Read the model definition and answer for the solid it produces. Units are mm, in the model's axes. A direction names the side the tool comes from. Coordinates: 2 decimals unless noted, no trailing zeros. Write each loop counter-clockwise with the first axis right and the second up, starting at its lowest first coordinate (ties: lowest second). Pieces come first, ordered by that corner, then holes. Notation, with made-up numbers: (-18, -39) - (-12, -39) arc R21 cw to (-12, -22) - close; hole circle Ø2 at (18, 82.5). An arc over 180 degrees is marked (long way). Return JSON: item names as keys, results as strings.
```python
from build123d import *

# Parameters (mm, degrees)
SKETCH_1_W          = 160
SKETCH_1_H          = 70
EXTRUDE_1_DEPTH     = 180
SHELL_1_T           = -10
SKETCH_2_W          = 3
SKETCH_2_H          = 70
EXTRUDE_2_DEPTH     = 170
CUT_EXTRUDE_1_DEPTH = 170
CUT_EXTRUDE_2_DEPTH = 170
CUT_EXTRUDE_3_REACH = 245.362
SKETCH_6_W          = 160
SKETCH_6_H          = 10
EXTRUDE_3_DEPTH     = 10
FILLET_1_R          = 3


with BuildPart() as part:
    # 草图1 → 凸台-拉伸1 (new body)
    with BuildSketch(Plane(origin=(0, 0, 0), x_dir=(1, 0, 0), z_dir=(0, 1, 0))):
        Rectangle(SKETCH_1_W, SKETCH_1_H)
    extrude(amount=EXTRUDE_1_DEPTH)

    # 抽壳1
    shell_1_openings = [part.faces().sort_by_distance(p)[0] for p in [
        (0, 90, 35),
    ]]
    offset(amount=SHELL_1_T, openings=shell_1_openings, kind=Kind.INTERSECTION)

    # 草图2 → 凸台-拉伸2 (add)
    with BuildSketch(Plane.XZ):
        with Locations((31.5, 0)):
            Rectangle(SKETCH_2_W, SKETCH_2_H)
        with Locations((28.5, 0)):
            Rectangle(SKETCH_2_W, SKETCH_2_H)
    extrude(amount=-EXTRUDE_2_DEPTH)

    # 草图3 → 切除-拉伸1 (cut)
    with BuildSketch(Plane.XY.offset(-25)):
        with BuildLine():
            Line((-8, 140), (-8, 40))
            ThreePointArc((-8, 40), (-21.5, 26.5), (-35, 40))
            Line((-35, 40), (-35, 140))
            ThreePointArc((-35, 140), (-21.5, 153.5), (-8, 140))
        make_face()
    extrude(amount=-CUT_EXTRUDE_1_DEPTH, mode=Mode.SUBTRACT)

    # 草图4 → 切除-拉伸2 (cut)
    with BuildSketch(Plane.XY.offset(-25)):
        with BuildLine():
            Line((59, 137.5), (59, 42.5))
            ThreePointArc((59, 42.5), (51.5, 35), (44, 42.5))
            Line((44, 42.5), (44, 137.5))
            ThreePointArc((44, 137.5), (51.5, 145), (59, 137.5))
        make_face()
    extrude(amount=-CUT_EXTRUDE_2_DEPTH, mode=Mode.SUBTRACT)

    # 草图5 → 切除-拉伸3 (cut, up to next)
    with BuildSketch(Plane.ZY.offset(80), mode=Mode.PRIVATE) as cut_extrude_3_sk1:
        with BuildLine():
            Line((-9.5, 165), (9.5, 165))
            ThreePointArc((9.5, 165), (12.328427125, 163.828427125), (13.5, 161))
            Line((13.5, 161), (13.5, 19))
            ThreePointArc((13.5, 19), (12.328427125, 16.171572875), (9.5, 15))
            Line((9.5, 15), (-9.5, 15))
            ThreePointArc((-9.5, 15), (-12.328427125, 16.171572875), (-13.5, 19))
            Line((-13.5, 19), (-13.5, 161))
            ThreePointArc((-13.5, 161), (-12.328427125, 163.828427125), (-9.5, 165))
        make_face()
    cut_extrude_3_tool1 = extrude(cut_extrude_3_sk1.sketch, amount=-CUT_EXTRUDE_3_REACH, mode=Mode.PRIVATE) & part.part
    add(cut_extrude_3_tool1.solids().sort_by_distance((-80, 90, 0))[0], mode=Mode.SUBTRACT)

    # 草图6 → 凸台-拉伸3 (add)
    with BuildSketch(Plane(origin=(0, 0, -35), x_dir=(-1, 0, 0), z_dir=(0, 0, -1))):
        with Locations((0, 5)):
            Rectangle(SKETCH_6_W, SKETCH_6_H)
    extrude(amount=EXTRUDE_3_DEPTH)

    # 圆角1
    fillet_1_edges = [part.edges().sort_by_distance(p)[0] for p in [
        (80, 5, -45),
        (0, 0, -45),
        (-80, 5, -45),
        (0, 10, -45),
    ]]
    fillet(fillet_1_edges, radius=FILLET_1_R)


solid = part.part
```
(1) Determine the mould class of faces 5 (the face through (80, 89, -3)), 6 (the face through (-75.07, 163.797, -12.359)), 7 (the face through (1, 10, -38)) for opening direction Y: +Y half, -Y half, draft (parallel to the pull), parting line (faces both ways), or undercut.
Answer:
{"face 5": "draft", "face 6": "undercut", "face 7": "+Y half"}
(2) A cutting plane is placed at C-C (z = -28.5). Determine the outline of the cut face in (x, y), and give its area (3 significant figures).
Answer:
{"outline": "(-80, 0) - (80, 0) - (80, 180) - (-80, 180) - close; hole (-35, 40) arc R13.5 ccw to (-8, 40) - (-8, 140) arc R13.5 ccw to (-35, 140) - close; hole (44, 42.5) arc R7.5 ccw to (59, 42.5) - (59, 137.5) arc R7.5 ccw to (44, 137.5) - close", "area": "23,900 mm²"}
(3) Flat-ended cylindrical pins translate along their axes: P1, Ø3.5, axis at x = -11.5, z = -39, coming from the +Y side; P2, Ø1, axis at x = -14, z = 9, coming from the -Y side; P3, Ø1, axis at x = 16.5, y = 111, coming from the -Z side; P4, Ø18.5, axis at x = 47.5, y = 60.5, coming from the +Z side. Find the tip coordinate at first contact, or state that the pin passes through.
Answer:
{"P1": "y = 10", "P2": "y = 0", "P3": "z = -35", "P4": "z = -25"}
(4) A cutting plane is placed at A-A (y = 131). Determine the outline of the cut face in (x, z), and give its area (3 significant figures).
Answer:
{"outline": "(-80, -35) - (-35, -35) - (-35, -25) - (-70, -25) - (-70, -13.5) - (-80, -13.5) - close; (-80, 13.5) - (-70, 13.5) - (-70, 35) - (-80, 35) - close; (-8, -35) - (44, -35) - (44, -25) - (33, -25) - (33, 35) - (27, 35) - (27, -25) - (-8, -25) - close; (59, -35) - (80, -35) - (80, 35) - (70, 35) - (70, -25) - (59, -25) - close", "area": "2,470 mm²"}
(5) A cutting plane is placed at B-B (x = -21.5). Determine the outline of the cut face in (y, z), and give its area (3 significant figures).
Answer:
{"outline": "(0, -42) arc R3 ccw to (3, -45) - (7, -45) arc R3 ccw to (10, -42) - (10, -35) - (26.5, -35) - (26.5, -25) - (10, -25) - (10, 35) - (0, 35) - close; (153.5, -35) - (180, -35) - (180, 35) - (170, 35) - (170, -25) - (153.5, -25) - close", "area": "1,830 mm²"}
(6) Straight lines are drawn through the part: line 1 (X direction, y = 101, z = -33); line 2 (X direction, y = 13.5, z = -1); line 3 (Y direction, x = 61, z = 5.5). For each, find the intervals that lie inside material, in ascending order. Write a range as from..to.
Answer:
{"line 1": "-80..-35, -8..44, 59..80", "line 2": "-80..-70, 27..33, 70..80", "line 3": "0..10, 170..180"}
(7) A cutting plane is placed at D-D (y = 151). Determine the outline of the cut face in (x, z), and give its area (3 significant figures).
Answer:
{"outline": "(-80, -35) - (-29.33, -35) - (-29.33, -25) - (-70, -25) - (-70, -13.5) - (-80, -13.5) - close; (-80, 13.5) - (-70, 13.5) - (-70, 35) - (-80, 35) - close; (-13.67, -35) - (80, -35) - (80, 35) - (70, 35) - (70, -25) - (33, -25) - (33, 35) - (27, 35) - (27, -25) - (-13.67, -25) - close", "area": "2,730 mm²"}
(8) Which of the six approach directions +Z, -Z, +X, -X, +Y, -Y give full straight-line access (tool end or side, diameter ignored) to faces 1 (the face through (33, 89, 5)), 2 (the face through (29, 83, 35)), 3 (the face through (-75.07, 16.141, -12.297)), 4 (the face through (51.34, 145, -29.93))?
Answer:
{"face 1": "+Z", "face 2": "+Z, +X, -X, +Y, -Y", "face 3": "-X", "face 4": "+Z, -Z"}
